Geometry check sheet. Reference: the model listing, model coordinates, mm. A direction names the side the tool comes from. Give positions to 0.01 mm unless a question says otherwise; leave off trailing zeros. Loops run counter-clockwise (first coordinate to the right, second up) from the corner with the lowest first, then second, coordinate; pieces in that order, holes last.
```python
from build123d import *

# Parameters (mm, degrees)
F0_W     = 25.4
F0_H     = 28.575
F1_DEPTH = 25.4


with BuildPart() as f1:
    # F0 (on Front) → F1 (new body)
    with BuildSketch(Plane.XZ):
        with BuildLine():
            add(Edge.make_bspline(
                [(-75.842815, 0), (-64.44554, 43.440532), (-15.861409, 53.869586), (22.582185, 52.4002)],
                knots=[0, 0, 0, 0, 111.504536, 111.504536, 111.504536, 111.504536], degree=3))
            Line((-75.842815, 0), (-12.342815, 0))
            Line((-12.342815, 0), (-12.342815, 17.4752))
            ThreePointArc((-12.342815, 17.4752), (-2.113519, 42.170904), (22.582185, 52.4002))
        make_face()
        Polygon((-12.342815, 0), (-75.842815, 0), (-75.842815, -19.05), (6.707185, -19.05), (6.707185, 0), align=None)
        with BuildLine():
            Line((-12.342815, 17.4752), (-12.342815, 0))
            Line((-12.342815, 0), (6.707185, 0))
            Line((6.707185, 0), (6.707185, 17.4752))
            ThreePointArc((6.707185, 17.4752), (11.356865, 28.70052), (22.582185, 33.3502))
            Line((22.582185, 33.3502), (31.884942, 33.3502))
            Line((31.884942, 33.3502), (31.884942, 52.4002))
            Line((31.884942, 52.4002), (22.582185, 52.4002))
            ThreePointArc((22.582185, 52.4002), (-2.113519, 42.170904), (-12.342815, 17.4752))
        make_face()
        Polygon((31.884942, 57.15), (31.884942, 52.4002), (31.884942, 33.3502), (31.884942, 28.575), (57.284942, 28.575), (57.284942, 57.15), align=None)
        with Locations((69.984942, 42.8625)):
            Rectangle(F0_W, F0_H)
    extrude(amount=F1_DEPTH)


solid = f1.part
```
1) Tool access check on faces 4 (the cylindrical face through (11.234, -12.522, 28.576)), 5 (the flat face through (82.685, -13, 43)), 6 (the flat face through (57, -13, 28.575)), 7 (the flat face through (-35, -13, -19.05)), 8 (the flat face through (27, -13, 52.4)). Record the directions out of +Z, -Z, +X, -X, +Y, -Y that give a thin tool (end or side, any length) a straight path to the whole face; none if there is none.
2) Scan lines: line 1 along Z through (x, y) = (37, -1.25) (3 decimals); line 2 along X through (y, z) = (-20.5, 31); line 3 along Z through (x, y) = (24, -18.5). Record each from-to range of solid material in increasing order.
3) Mould release check, pull along X, two halves, no side actions. Record for faces 1 (the flat face through (6.707, -13, -1)), 2 (the flat face through (31.885, -13, 31)), 3 (the flat face through (-13, 0, 20)): +X half, -X half, draft (parallel to the pull), parting line (faces both ways), or undercut.
4) Sectioned sample at A-A on x = 41.5. Enter the section's corners in (y, z) (3 decimals).
5) Depth check by flat-ended pin: P1, Ø4, axis at y = -11.5, z = 55.5, coming from the -X side; P2, Ø2, axis at y = -8, z = -9.5, coming from the +X side; P3, Ø2.5, axis at y = -18.5, z = 32, coming from the -X side. Enter the tip coordinate at first touch or a pass-through.
6) Sectioned sample at B-B on z = -7. Enter the section's corners in (x, y).
Determined:
1. face 4: -Z, +Y, -Y
1. face 5: +Z, -Z, +X, +Y, -Y
1. face 6: -Z, +X, +Y, -Y
1. face 7: -Z, +X, -X, +Y, -Y
1. face 8: +Z, +Y, -Y
2. line 1: z = 28.575 to 57.15
2. line 2: x = -56.54 to 14.27, 31.88 to 82.68
2. line 3: z = 33.35 to 52.4
3. face 1: +X half
3. face 2: undercut
3. face 3: draft
4. outline: (-25.4, 28.575) - (0, 28.575) - (0, 57.15) - (-25.4, 57.15) - close
5. P1: stops at x = 31.88
5. P2: stops at x = 6.71
5. P3: stops at x = -56.83
6. outline: (-75.84, -25.4) - (6.71, -25.4) - (6.71, 0) - (-75.84, 0) - close
